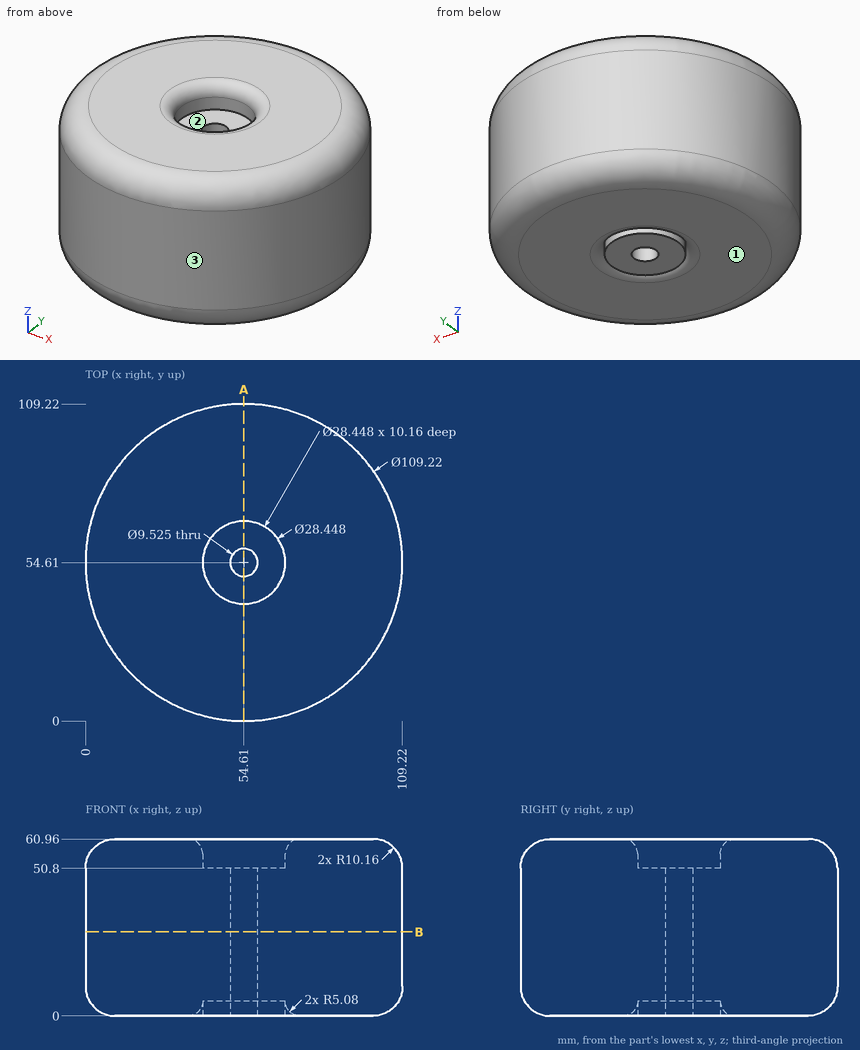
Geometry check sheet. Reference: drawing and pictorial views, mm from the part's lowest x, y, z. Coordinates: 2 decimals unless noted, no trailing zeros. Loops run counter-clockwise (first coordinate to the right, second up) from the corner with the lowest first, then second, coordinate; pieces in that order, holes last. Notation, with made-up numbers: (-2, 17.5) - (23, 17.5) arc R18 ccw to (23, 50.5) - close; hole circle Ø8 at (78, 2). An arc over 180 degrees is marked (long way). Return JSON: item names as keys, results as strings.
1. Section check A-A, the plane x = 54.61. Record the boundary of the cut face in (y, z), then the cut area to 3 significant figures.
Established:
{"outline": "(0, 10.16) arc R10.16 ccw to (10.16, 0) - (35.31, 0) arc R5.08 ccw to (40.39, 5.08) - (40.39, 0) - (49.85, 0) - (49.85, 50.8) - (40.39, 50.8) - (40.39, 55.88) arc R5.08 ccw to (35.31, 60.96) - (10.16, 60.96) arc R10.16 ccw to (0, 50.8) - close; (59.37, 0) - (68.83, 0) - (68.83, 5.08) arc R5.08 ccw to (73.91, 0) - (99.06, 0) arc R10.16 ccw to (109.22, 10.16) - (109.22, 50.8) arc R10.16 ccw to (99.06, 60.96) - (73.91, 60.96) arc R5.08 ccw to (68.83, 55.88) - (68.83, 50.8) - (59.37, 50.8) - close", "area": "5,770 mm2"}
2. Mould release check, pull along X, two halves, no side actions. Record for the marked faces 1, 2 and 3: +X half, -X half, draft (parallel to the pull), parting line (faces both ways), or undercut.
Established:
{"face 1": "draft", "face 2": "undercut", "face 3": "parting line"}
3. Thickness scan on L1, parallel to Y at x = 54.61, z = 22.5; L2, parallel to Y at x = 54, z = 53; L3, parallel to X at y = 58.5, z = 37. Record the ranges inside material, lowest first.
Established:
{"L1": "y = 0 to 49.85, 59.37 to 109.22", "L2": "y = 0.24 to 40.4, 68.82 to 108.98", "L3": "x = 0.14 to 51.86, 57.36 to 109.08"}
4. Go/stop test with flat-tipped pins: pin 1 (8.5 mm diameter, centred on x = 56.5, y = 50, fed in from +Z); pin 2 (8 mm diameter, centred on y = 16, z = 52, fed in from -X); pin 3 (4 mm diameter, centred on y = 24.5, z = 44, fed in from +X); pin 4 (5.5 mm diameter, centred on x = 54.61, y = 54.61, fed in from -Z). Record where each tip stops, or that it passes through.
Established:
{"pin 1": "stops at z = 50.8", "pin 2": "stops at x = 12.42", "pin 3": "stops at x = 101.43", "pin 4": "passes through"}
5. Section check B-B, the plane z = 29. Record the boundary of the cut face in (x, y) (1 decimal).
Established:
{"outline": "circle Ø109.2 at (54.6, 54.6); hole circle Ø9.5 at (54.6, 54.6)"}
